from build123d import *

# Parameters (mm, degrees)
F1_DEPTH = 25.908
F2_DEPTH = 10.668
F3_W     = 16.764
F3_H     = 8.548961
F4_DEPTH = 83.312


with BuildPart() as f1:
    # F0 (on Front) → F1 (new body, symmetric)
    with BuildSketch(Plane.XZ):
        Polygon((34.290001, -52.7304), (34.290001, 0), (22.707598, 0), (22.707598, -41.452803), (-28.8036, -41.452803), (-28.8036, -27.432), (-45.262802, -27.432), (-45.262802, -52.7304), align=None)
    extrude(amount=F1_DEPTH, both=True)

    # F0 (on Front) → F2 (join, symmetric)
    with BuildSketch(Plane.XZ):
        Polygon((22.707598, -41.452803), (22.707598, 0), (0, 0), (-28.8036, -27.432), (-28.8036, -41.452803), align=None)
    extrude(amount=F2_DEPTH, both=True)

    # F3 (on face) → F4 (cut)
    with BuildSketch(Plane.YZ.offset(34.290001)):
        with Locations((0, -8.534401)):
            Rectangle(F3_W, F3_H)
    extrude(amount=-F4_DEPTH, mode=Mode.SUBTRACT)


solid = f1.part
Could you check a few things on this model? Use its own coordinates, in mm. A direction names the side the tool comes from. Coordinates: 2 decimals unless noted, no trailing zeros. Order: outer loops, then holes, each group sorted by start corner. A loop starts at its lowest first (then second) coordinate and runs counter-clockwise, first axis right, second up. Notation, with made-up numbers: (-28.5, -18.75) -> (30.5, -18.75) arc R31 ccw to (30.5, 19.25) -> close; hole circle Ø2 at (73.5, 8). An arc over 180 degrees is marked (long way). One line per question, with ' | ' between items.
Q1. Imagine slicing it at B-B on x = 27. Please give me the cut outline in (y, z).
Return value:
outline: (-25.91, -52.73) -> (25.91, -52.73) -> (25.91, 0) -> (-25.91, 0) -> close; hole (-8.38, -12.81) -> (8.38, -12.81) -> (8.38, -4.26) -> (-8.38, -4.26) -> close
Q2. If I drill on L1, parallel to Z at x = 22.5, y = -5.5; L2, parallel to Z at x = -26.5, y = -21.5; L3, parallel to X at y = 15, z = -15.5, over which ranges is the centre line in solid material (lowest first)?
Return value:
L1: -52.73 to -12.81, -4.26 to 0 | L2: -52.73 to -41.45 | L3: 22.71 to 34.29
Q3. Imagine slicing it at D-D on y = 17.5. Please give me the cut outline in (x, z).
Return value:
outline: (-45.26, -52.73) -> (34.29, -52.73) -> (34.29, 0) -> (22.71, 0) -> (22.71, -41.45) -> (-28.8, -41.45) -> (-28.8, -27.43) -> (-45.26, -27.43) -> close
Q4. On a 3-axis mill with a long thin cutter (end or side, diameter ignored), from which of +Z, -Z, +X, -X, +Y, -Y can I reach the whole of each face in a straight line? I mean faces 5 (the face through (22.708, -18, -20)), 6 (the face through (2, 10.668, -25)), 7 (the face through (15, 0, -4.26)). Say none if no direction works.
Return value:
face 5: +Z, -Y | face 6: +Z, +Y | face 7: +X, -X
Q5. Imagine slicing it at A-A on y = -7. Please give me the cut outline in (x, z).
Return value:
outline: (-45.26, -52.73) -> (34.29, -52.73) -> (34.29, -12.81) -> (-13.45, -12.81) -> (-28.8, -27.43) -> (-45.26, -27.43) -> close; (-4.47, -4.26) -> (34.29, -4.26) -> (34.29, 0) -> (0, 0) -> close
Q6. I'm going to push flat-ended pins straight in: P1, Ø3, axis at x = 2.5, z = -10, coming from the +Y side; P2, Ø2.5, axis at x = 13, z = -10.5, coming from the -Y side; P3, Ø6, axis at x = 0, y = 5, coming from the +Z side; P4, Ø7.5, axis at y = 14.5, z = -13.5, coming from the -X side. Where does each tip first touch, or does it pass through?
Return value:
P1: y = 10.67 | P2: y = -10.67 | P3: z = 0 | P4: x = 22.71
Q7. Thinking about a two-plate mould opening in Z: for faces 1 (the face through (-37, 0, -27.432)), 2 (the face through (11, 0, -12.809)), 3 (the face through (34.29, 0, -27)), 4 (the face through (11, -8.382, -9)), which applies, pulls with the +Z half, pulls with the -Z half, needs draft (parallel to the pull), parting line crosses it, or undercut?
Return value:
face 1: pulls with the +Z half | face 2: undercut | face 3: needs draft | face 4: undercut
Q8. Imagine slicing it at C-C on z = -11. Please give me the cut outline in (x, y), and give its area (3 significant figures).
Return value:
outline: (-11.55, -10.67) -> (22.71, -10.67) -> (22.71, -25.91) -> (34.29, -25.91) -> (34.29, -8.38) -> (-11.55, -8.38) -> close; (-11.55, 8.38) -> (34.29, 8.38) -> (34.29, 25.91) -> (22.71, 25.91) -> (22.71, 10.67) -> (-11.55, 10.67) -> close | area: 563 mm²
